Here's how the part is built. I have some questions about the finished solid (model axes, mm). Give positions to 0.01 mm unless a question says otherwise; leave off trailing zeros. Order: outer loops, then holes, each group sorted by start corner. A loop starts at its lowest first (then second) coordinate and runs counter-clockwise, first axis right, second up. Notation, with made-up numbers: M 72.25,-23 L 131.25,-23 A22 ccw 131.25,-12 Z; hole C 82,-40 d8. An arc over 180 degrees is marked long. Use one line per item in the form item = value.
from build123d import *

# Parameters (mm, degrees)
ESBO_O1_R                = 1.25
ESBO_O1_R_2              = 1.6
RESSALTO_EXTRUS_O1_DEPTH = 1
FILETE1_R                = 3


with BuildPart() as part:
    # Esboço1 → Ressalto-extrusão1 (new body)
    with BuildSketch(Plane.XY):
        Polygon((-9, 9.5), (9, 9.5), (36.5, 9.5), (36.5, -5.5), (9, -9.5), (-9, -9.5), align=None)
        with Locations((6, -6.5)):
            Circle(ESBO_O1_R, mode=Mode.SUBTRACT)
        with Locations((6, 6.5)):
            Circle(ESBO_O1_R, mode=Mode.SUBTRACT)
        with Locations((-6, -6.5)):
            Circle(ESBO_O1_R, mode=Mode.SUBTRACT)
        with Locations((-6, 6.5)):
            Circle(ESBO_O1_R, mode=Mode.SUBTRACT)
        with Locations((31.5, 2)):
            Circle(ESBO_O1_R_2, mode=Mode.SUBTRACT)
        with Locations((14, 2)):
            Circle(ESBO_O1_R_2, mode=Mode.SUBTRACT)
    extrude(amount=RESSALTO_EXTRUS_O1_DEPTH)

    # Filete1
    filete1_edges = [part.edges().sort_by_distance(p)[0] for p in [
        (9, -9.5, 0.5),
        (-9, -9.5, 0.5),
        (-9, 9.5, 0.5),
        (36.5, 9.5, 0.5),
        (36.5, -5.5, 0.5),
    ]]
    fillet(filete1_edges, radius=FILETE1_R)


solid = part.part
Q1. I want a section at D-D on x = 14. Write out the boundary of the cut face in (y, z).
Found:
outline = M -8.77,0 L 0.4,0 L 0.4,1 L -8.77,1 Z; M 3.6,0 L 9.5,0 L 9.5,1 L 3.6,1 Z
Q2. I'm going to push a flat-ended pin straight in: pin 1 Ø4 at (x, y) = (13, -6.5) entering from -Z. Where does the tip first touch, or does it pass through?
Found:
pin_1 = 0
Q3. I want a section at C-C on x = 31.5. Write out the boundary of the cut face in (y, z).
Found:
outline = M -6.23,0 L 0.4,0 L 0.4,1 L -6.23,1 Z; M 3.6,0 L 9.5,0 L 9.5,1 L 3.6,1 Z
Q4. I need wall thicknesses on L1, parallel to Y at x = 6, z = 0.8; L2, parallel to X at y = 3.25, z = 0.55; L3, parallel to X at y = 6, z = 0.3. Which ranges of each line are inside material? Lowest first, please.
Found:
L1 = -9.5 to -7.75, -5.25 to 5.25, 7.75 to 9.5
L2 = -9 to 13, 15 to 30.5, 32.5 to 36.5
L3 = -9 to -7.15, -4.85 to 4.85, 7.15 to 36.5
Q5. I want a section at A-A on z = 0.65. Write out the boundary of the cut face in (x, y).
Found:
outline = M -9,-6.5 A3 ccw -6,-9.5 L 8.78,-9.5 A3 ccw 9.21,-9.47 L 33.93,-5.87 A3 ccw 36.5,-2.9 L 36.5,6.5 A3 ccw 33.5,9.5 L -6,9.5 A3 ccw -9,6.5 Z; hole C -6,-6.5 d2.5; hole C -6,6.5 d2.5; hole C 6,-6.5 d2.5; hole C 6,6.5 d2.5; hole C 14,2 d3.2; hole C 31.5,2 d3.2
Q6. I want a section at B-B on x = 6. Write out the boundary of the cut face in (y, z), then the cut area to 3 significant figures.
Found:
outline = M -9.5,0 L -7.75,0 L -7.75,1 L -9.5,1 Z; M -5.25,0 L 5.25,0 L 5.25,1 L -5.25,1 Z; M 7.75,0 L 9.5,0 L 9.5,1 L 7.75,1 Z
area = 14.0 mm²
Q7. Thinking about a two-plate mould opening in X: for faces 1 (the face through (1.5, -9.5, 0.5)), 2 (the face through (-9, -0.1, 0.5)), 3 (the face through (29.9, 2.07, 0.49)), which applies, +X half, -X half, draft (parallel to the pull), parting line (faces both ways), or undercut?
Found:
face_1 = draft
face_2 = -X half
face_3 = undercut
